Design review of the part shown in the three views and the two pictorial views. Dimensions are in mm from the part's minimum x, y and z. A direction names the side the tool comes from. Coordinates: 2 decimals unless noted, no trailing zeros. Loops run counter-clockwise (first coordinate to the right, second up) from the corner with the lowest first, then second, coordinate; pieces in that order, holes last.
Q1. Add section A-A on y = 7. Give the boundary of the cut face in (x, z).
Q2. Add section B-B on x = 39. Give the boundary of the cut face in (y, z), and give its area (3 significant figures).
Q3. Machinability: for the marked faces 1, 2 and 3, which of the approach directions +Z, -Z, +X, -X, +Y, -Y give a long, thin tool a straight path to every point of the face, cutting with its end or side? Answer none if there is none.
Q4. Add section C-C on z = 17. Give the boundary of the cut face in (x, y).
Q5. Draft analysis for pull direction X (two halves, no side actions). For the marked faces 4, 5 and 6, state which applies: released by +X, released by -X, zero draft, split by the parting line, or undercut.
Q6. For P1, Ø2.5, axis at x = 28.5, y = 41.5, coming from the -Z side; P2, Ø3, axis at x = 14, y = 37, coming from the -Z side, all flat-tipped, find the tip position at first contact; note any pin that passes through.
Q7. Wall thickness on probe 1 along Y at (x, z) = (17.5, 7.25); probe 2 along X at (y, z) = (18, 7); probe 3 along Z at (x, y) = (41, 14): over which ranges is each line inside the solid? List them lowest first.
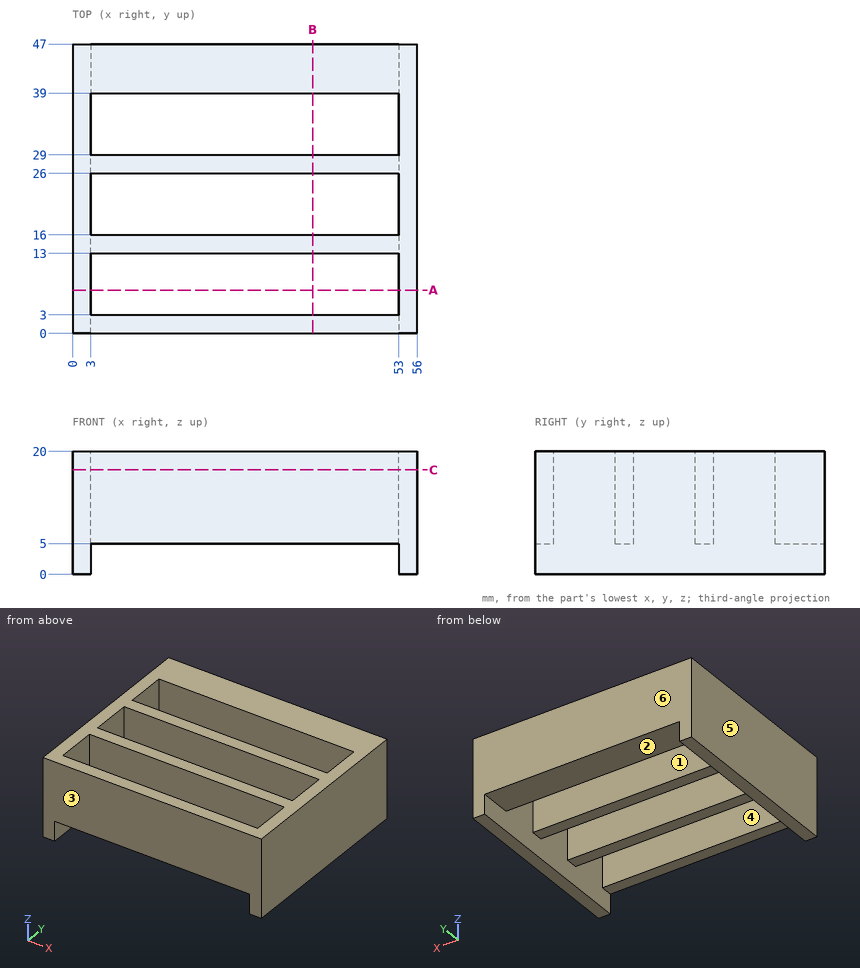
Entries:
1. outline: (0, 0) - (3, 0) - (3, 20) - (0, 20) - close; (53, 0) - (56, 0) - (56, 20) - (53, 20) - close
2. outline: (0, 5) - (3, 5) - (3, 20) - (0, 20) - close; (13, 5) - (16, 5) - (16, 20) - (13, 20) - close; (26, 5) - (29, 5) - (29, 20) - (26, 20) - close; (39, 5) - (47, 5) - (47, 20) - (39, 20) - close
2. area: 255 mm2
3. face 1: +Z, -Z
3. face 2: -Z, +Y, -Y
3. face 3: +Z, -Z, +X, -X, -Y
4. outline: (0, 0) - (56, 0) - (56, 47) - (0, 47) - close; hole (3, 3) - (53, 3) - (53, 13) - (3, 13) - close; hole (3, 16) - (53, 16) - (53, 26) - (3, 26) - close; hole (3, 29) - (53, 29) - (53, 39) - (3, 39) - close
5. face 4: undercut
5. face 5: released by -X
5. face 6: zero draft
6. P1: stops at z = 5
6. P2: passes through
7. probe 1: y = 0 to 3, 13 to 16, 26 to 29, 39 to 47
7. probe 2: x = 0 to 3, 53 to 56
7. probe 3: z = 5 to 20
